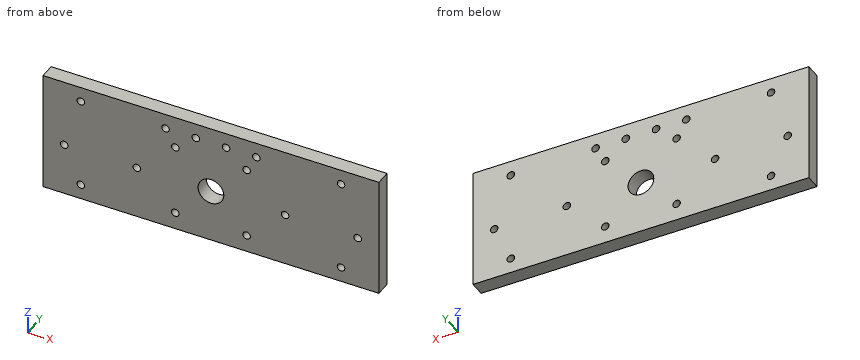
```python
from build123d import *

# Parameters (mm, degrees)
F0_W     = 222
F0_H     = 80
F1_DEPTH = 10
F2_D     = 5
F3_D     = 17
F4_D     = 5
F5_D     = 5
F6_D     = 5


with BuildPart() as f1:
    # F0 (on Front) → F1 (new body)
    with BuildSketch(Plane.XZ):
        Rectangle(F0_W, F0_H)
    extrude(amount=F1_DEPTH)

    # F2 (through all)
    with Locations(Plane(origin=(0, 0, 0), x_dir=(1, 0, 0), z_dir=(0, 1, 0))):
        with Locations((97, 5), (49, 5), (-49, 5), (-97, 5)):
            Hole(F2_D / 2)

    # F3 (through all)
    with Locations(Plane(origin=(0, 0, 0), x_dir=(1, 0, 0), z_dir=(0, 1, 0))):
        with Locations((0, 5)):
            Hole(F3_D / 2)

    # F4 (through all)
    with Locations(Plane(origin=(0, 0, 0), x_dir=(1, 0, 0), z_dir=(0, 1, 0))):
        with Locations((-86, -30), (-86, 30), (86, 30), (86, -30)):
            Hole(F4_D / 2)

    # F5 (through all)
    with Locations(Plane(origin=(0, 0, 0), x_dir=(1, 0, 0), z_dir=(0, 1, 0))):
        with Locations((-30, -30), (-10, -30), (10, -30), (30, -30)):
            Hole(F5_D / 2)

    # F6 (through all)
    with Locations(Plane(origin=(0, 0, 0), x_dir=(1, 0, 0), z_dir=(0, 1, 0))):
        with Locations((-23.57, -18.57), (23.57, -18.57), (23.57, 28.57), (-23.57, 28.57)):
            Hole(F6_D / 2)


solid = f1.part
```
Can you work these out from the model? Positions are in its coordinate system, mm. Round coordinates to 2 decimals unless told otherwise and drop trailing zeros. Loops run counter-clockwise (first coordinate to the right, second up) from the corner with the lowest first, then second, coordinate; pieces in that order, holes last.
Item 1: Suppose I cut it at B-B, the plane y = -5.5. State how many separate pieces and enclosed holes the cut face has, then the cut area to 3 significant figures.
Item 2: Suppose I cut it at D-D, the plane x = 0. Write out the boundary of the cut face in (y, z), then the cut area to 3 significant figures.
Item 3: Suppose I cut it at C-C, the plane x = 97. Write out the boundary of the cut face in (y, z), then the cut area to 3 significant figures.
Item 4: Suppose I cut it at A-A, the plane z = -5. Write out the boundary of the cut face in (x, y), then the cut area to 3 significant figures.
Item 5: Will this pin go through, and if not, where does the flat tip stop? pin 1 Ø3 at (x, z) = (-86, -30) entering from -Y.
Item 6: Please list where these lines run through material, in increasing order: L1, parallel to X at y = -2.5, z = 18.57; L2, parallel to Z at x = -86, y = -5; L3, parallel to Z at x = 23, y = -8.
Reported:
1. separate pieces: 1
1. enclosed holes: 17
1. area: 17,200 mm2
2. outline: (-10, -40) - (0, -40) - (0, -13.5) - (-10, -13.5) - close; (-10, 3.5) - (0, 3.5) - (0, 40) - (-10, 40) - close
2. area: 630 mm2
3. outline: (-10, -40) - (0, -40) - (0, -7.5) - (-10, -7.5) - close; (-10, -2.5) - (0, -2.5) - (0, 40) - (-10, 40) - close
3. area: 750 mm2
4. outline: (-111, -10) - (-99.5, -10) - (-99.5, 0) - (-111, 0) - close; (-94.5, -10) - (-51.5, -10) - (-51.5, 0) - (-94.5, 0) - close; (-46.5, -10) - (-8.5, -10) - (-8.5, 0) - (-46.5, 0) - close; (8.5, -10) - (46.5, -10) - (46.5, 0) - (8.5, 0) - close; (51.5, -10) - (94.5, -10) - (94.5, 0) - (51.5, 0) - close; (99.5, -10) - (111, -10) - (111, 0) - (99.5, 0) - close
4. area: 1,850 mm2
5. pin 1: passes through
6. L1: x = -111 to -26.07, -21.07 to 21.07, 26.07 to 111
6. L2: z = -40 to -32.5, -27.5 to 27.5, 32.5 to 40
6. L3: z = -40 to -31, -26.14 to 16.14, 21 to 40
